Source: three-view drawing plus pictorial views. Frame: mm from the lowest corner of the part. A direction names the side the tool comes from. Coordinates: 2 decimals unless noted, no trailing zeros. Write each loop counter-clockwise with the first axis right and the second up, starting at its lowest first coordinate (ties: lowest second). Pieces come first, ordered by that corner, then holes. Notation, with made-up numbers: (37, 29.5) - (80, 29.5) arc R12 cw to (80, 41.5) - close; hole circle Ø9 at (28.5, -17). An arc over 180 degrees is marked (long way). One line per item, written item: value.
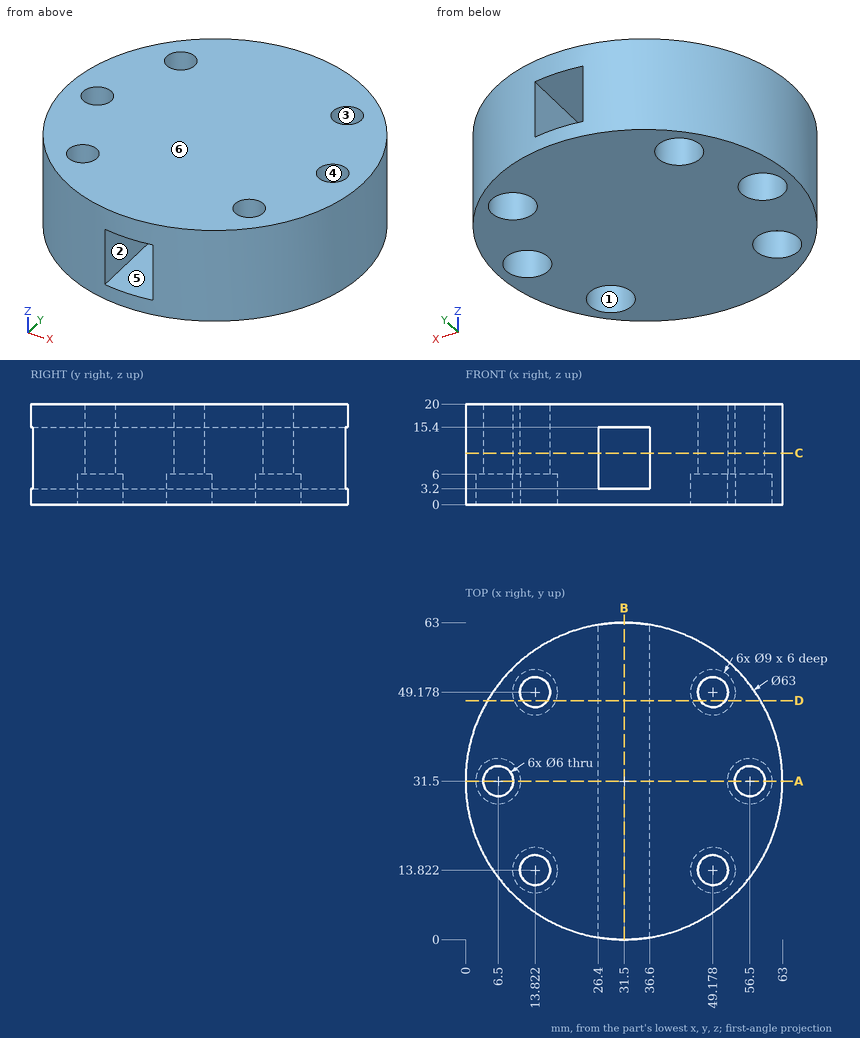
1) Section query D-D on y = 47.5. Output: boundary loops of the cut face in (x, z) (1 decimal).
Values found:
outline: (4.4, 0) - (9.6, 0) - (9.6, 6) - (11.3, 6) - (11.3, 20) - (4.4, 20) - close; (16.3, 6) - (18, 6) - (18, 0) - (45, 0) - (45, 6) - (46.7, 6) - (46.7, 20) - (16.3, 20) - close; (51.7, 6) - (53.4, 6) - (53.4, 0) - (58.6, 0) - (58.6, 20) - (51.7, 20) - close; hole (26.4, 3.2) - (36.6, 3.2) - (36.6, 15.4) - (26.4, 15.4) - close
2) Material intervals for line 1 (Y direction, x = 11.5, z = 16.5) (1 decimal); line 2 (X direction, y = 14, z = 7.25); line 3 (X direction, y = 16, z = 1.5) (1 decimal), sorted ascending.
Values found:
line 1: 7.2 to 11.9, 15.7 to 47.3, 51.1 to 55.8
line 2: 5.31 to 10.83, 16.82 to 26.4, 36.6 to 46.18, 52.17 to 57.69
line 3: 4.1 to 9.9, 17.8 to 45.2, 53.1 to 58.9
3) Draft query along Z for the marked faces 4, 5 and 6. Return one class per face: released by +Z, released by -Z, zero draft, split by the parting line, or undercut.
Values found:
face 4: zero draft
face 5: undercut
face 6: released by +Z
4) Contact query for flat-ended pins moving along their axis: P1, Ø5, axis at x = 49, y = 56, coming from the -Z side; P2, Ø4, axis at y = 47.5, z = 9, coming from the -X side; P3, Ø10, axis at y = 42, z = 9.5, coming from the -X side; P4, Ø3.5, axis at y = 25, z = 7.5, coming from the -X side. Output: stop coordinate, or through.
Values found:
P1: z = 0
P2: x = 3.28
P3: x = 0.48
P4: x = 0.36
5) Reachability of the marked faces 1, 2 and 3 from +Z, -Z, +X, -X, +Y, -Y: full face, straight path, thin tool, end or side. Return the list, or none.
Values found:
face 1: -Z
face 2: +Y, -Y
face 3: +Z, -Z
6) Section query B-B on x = 31.5. Output: boundary loops of the cut face in (y, z).
Values found:
outline: (0, 0) - (63, 0) - (63, 3.2) - (0, 3.2) - close; (0, 15.4) - (63, 15.4) - (63, 20) - (0, 20) - close
7) Section query A-A on y = 31.5. Output: boundary loops of the cut face in (x, z).
Values found:
outline: (0, 0) - (2, 0) - (2, 6) - (3.5, 6) - (3.5, 20) - (0, 20) - close; (9.5, 6) - (11, 6) - (11, 0) - (52, 0) - (52, 6) - (53.5, 6) - (53.5, 20) - (9.5, 20) - close; (59.5, 6) - (61, 6) - (61, 0) - (63, 0) - (63, 20) - (59.5, 20) - close; hole (26.4, 3.2) - (36.6, 3.2) - (36.6, 15.4) - (26.4, 15.4) - close
8) Section query C-C on z = 10.25. Output: boundary loops of the cut face in (x, y) (1 decimal).
Values found:
outline: (26.4, 0.4) - (26.4, 62.6) arc R31.5 ccw to start; (36.6, 0.4) arc R31.5 ccw to (36.6, 62.6) - close; hole circle Ø6 at (6.5, 31.5); hole circle Ø6 at (13.8, 13.8); hole circle Ø6 at (13.8, 49.2); hole circle Ø6 at (49.2, 13.8); hole circle Ø6 at (49.2, 49.2); hole circle Ø6 at (56.5, 31.5)
